Model file for the job. Use its own axes, mm. A direction names the side the tool comes from. Give positions to 0.01 mm unless a question says otherwise; leave off trailing zeros. Order: outer loops, then holes, each group sorted by start corner. A loop starts at its lowest first (then second) coordinate and runs counter-clockwise, first axis right, second up. Notation, with made-up numbers: (33.25, 9) -> (66.25, 9) arc R22 ccw to (66.25, 29) -> close; hole circle Ø1 at (-29, -19). An arc over 180 degrees is marked (long way). Answer in a Markdown table with one row per item. Add a question column.
from build123d import *

# Parameters (mm, degrees)
BOSS_EXTRUDE1_DEPTH     = 122.6
SKETCH2_W               = 52.856609426
SKETCH2_H               = 136.885065439
CUT_EXTRUDE1_DEPTH      = 1.4
CUT_EXTRUDE2_DEPTH      = 1
CUT_EXTRUDE2_DEPTH_BACK = 123.6


with BuildPart() as part:
    # Sketch1 → Boss-Extrude1 (new body)
    with BuildSketch(Plane(origin=(0, 0, 0), x_dir=(1, 0, 0), z_dir=(0, 1, 0))):
        Polygon((-4.75, 15), (-4.75, 5.05), (-14.75, 5.05), (-14.75, 6.4), (-91, 6.4), (-91, 0), (-32.25, 0), (-32.25, 2), (-31.25, 2), (-31.25, 0), (0, 0), (0, 15), align=None)
    extrude(amount=BOSS_EXTRUDE1_DEPTH)

    # Sketch2 → Cut-Extrude1 (cut)
    with BuildSketch(Plane(origin=(0, 0, 0), x_dir=(0, 0, -1), z_dir=(1, 0, 0))):
        with Locations((4.111755806, 55.794103185)):
            Rectangle(SKETCH2_W, SKETCH2_H)
    extrude(amount=-CUT_EXTRUDE1_DEPTH, mode=Mode.SUBTRACT)

    # Sketch3 → Cut-Extrude2 (cut, two sides)
    with BuildSketch(Plane(origin=(0, 122.6, 0), x_dir=(1, 0, 0), z_dir=(0, 1, 0))) as cut_extrude2_sk:
        Polygon((-1.4, 5.05), (-56.4, 5.05), (-60.82107113, 9.47107113), (-60.82107113, 21.013712959), (-1.4, 21.013712959), align=None)
    extrude(amount=CUT_EXTRUDE2_DEPTH, mode=Mode.SUBTRACT)
    extrude(cut_extrude2_sk.sketch, amount=-CUT_EXTRUDE2_DEPTH_BACK, mode=Mode.SUBTRACT)


solid = part.part
Item 1: Wall check: line 1 (X direction, y = 56, z = -1.25); line 2 (Z direction, x = -11, y = 93.5). Give the ranges that are in metal, low to high.
Item 2: Saw through at A-A on y = 73.5. List the corners of the cut face in (x, z).
Item 3: Saw through at B-B on x = -20.5. List the corners of the cut face in (y, z), plus the area to 3 significant figures.
Item 4: Which spindle directions (+Z, -Z, +X, -X, +Y, -Y) get a long thin tool onto all of the face, cutting with end or side? Do faces 1 (the flat face through (-91, 60, -3)), 2 (the flat face through (-29, 60, -5.05)). Say none if no direction does.
Evaluation:
| question | item | result |
|---|---|---|
| 1 | line 1 | x = -91 to -32.25, -31.25 to -1.4 |
| 1 | line 2 | z = -5.05 to 0 |
| 2 | outline | (-91, -6.4) -> (-57.75, -6.4) -> (-56.4, -5.05) -> (-1.4, -5.05) -> (-1.4, 0) -> (-31.25, 0) -> (-31.25, -2) -> (-32.25, -2) -> (-32.25, 0) -> (-91, 0) -> close |
| 3 | outline | (0, -5.05) -> (122.6, -5.05) -> (122.6, 0) -> (0, 0) -> close |
| 3 | area | 619 mm2 |
| 4 | face 1 | +Z, -Z, -X, +Y, -Y |
| 4 | face 2 | -Z, +X, +Y, -Y |
